```python
from build123d import *

# Parameters (mm, degrees)
F0_R         = 9.525
F1_DEPTH     = 25.4
F3_DEPTH     = 25.401
F4_DEPTH     = 11.0998
F6_DEPTH     = 5.08
F7_W         = 101.6
F7_H         = 127
F8_DEPTH     = 38.1
F9_T         = 2.54
F9_T3_DEPTH  = 10.16
F9_T5_DEPTH  = 11.43
F9_T7_DEPTH  = 11.43
F9_T9_DEPTH  = 11.43
F9_T11_DEPTH = 11.43
F9_T13_DEPTH = 11.43
F9_T15_DEPTH = 9.8425
F9_T17_DEPTH = 9.8425
F9_T19_DEPTH = 9.8425
F9_T21_DEPTH = 9.8425
F9_T23_DEPTH = 14.605
F9_T25_DEPTH = 16.1798
F9_T27_DEPTH = 14.605


# Not quite as in the source:
# - a shell that OpenCascade refuses in one call is made with other operations: the cavity is built on its own and cut out


with BuildPart() as f1:
    # F0 (on Front) → F1 (new body)
    with BuildSketch(Plane.XZ):
        Circle(F0_R)
    extrude(amount=F1_DEPTH)

    # F2 (on face) → F3 (cut, through all)
    with BuildSketch(Plane(origin=(0, 0, 0), x_dir=(-1, 0, 0), z_dir=(0, 1, 0))):
        with BuildLine():
            ThreePointArc((4.7625, 0), (3.3675960454, 3.3675960454), (0, 4.7625))
            ThreePointArc((0, 4.7625), (-3.3675960454, 3.3675960454), (-4.7625, 0))
            ThreePointArc((-4.7625, 0), (-3.3675960454, -3.3675960454), (0, -4.7625))
            ThreePointArc((0, -4.7625), (3.3675960454, -3.3675960454), (4.7625, 0))
        make_face()
    extrude(amount=-F3_DEPTH, mode=Mode.SUBTRACT)

    # F2 (on face) → F4 (cut)
    with BuildSketch(Plane(origin=(0, 0, 0), x_dir=(-1, 0, 0), z_dir=(0, 1, 0))):
        with BuildLine():
            Line((4.7625, 0), (4.7625, 4.7625))
            Line((4.7625, 4.7625), (0, 4.7625))
            ThreePointArc((0, 4.7625), (3.3675960454, 3.3675960454), (4.7625, 0))
        make_face()
        with BuildLine():
            ThreePointArc((-4.7625, 0), (-3.3675960454, 3.3675960454), (0, 4.7625))
            Line((0, 4.7625), (-4.7625, 4.7625))
            Line((-4.7625, 4.7625), (-4.7625, 0))
        make_face()
        with BuildLine():
            ThreePointArc((4.7625, 0), (3.3675960454, 3.3675960454), (0, 4.7625))
            ThreePointArc((0, 4.7625), (-3.3675960454, 3.3675960454), (-4.7625, 0))
            ThreePointArc((-4.7625, 0), (-3.3675960454, -3.3675960454), (0, -4.7625))
            ThreePointArc((0, -4.7625), (3.3675960454, -3.3675960454), (4.7625, 0))
        make_face()
        with BuildLine():
            Line((4.7625, -4.7625), (4.7625, 0))
            ThreePointArc((4.7625, 0), (3.3675960454, -3.3675960454), (0, -4.7625))
            Line((0, -4.7625), (4.7625, -4.7625))
        make_face()
        with BuildLine():
            ThreePointArc((0, -4.7625), (-3.3675960454, -3.3675960454), (-4.7625, 0))
            Line((-4.7625, 0), (-4.7625, -4.7625))
            Line((-4.7625, -4.7625), (0, -4.7625))
        make_face()
    extrude(amount=-F4_DEPTH, mode=Mode.SUBTRACT)

    # F5 (on face) → F6 (cut)
    with BuildSketch(Plane.XZ.offset(25.4)):
        Polygon((3.175, 5.499261314), (-3.175, 5.499261314), (-6.35, 0), (-3.175, -5.499261314), (3.175, -5.499261314), (6.35, 0), align=None)
    extrude(amount=-F6_DEPTH, mode=Mode.SUBTRACT)

    # F7 (on Front) → F8 (join)
    with BuildSketch(Plane.XZ):
        Rectangle(F7_W, F7_H)
    extrude(amount=-F8_DEPTH)

    # F9: shell of thickness 2.54, made by hand


with BuildPart() as f9_core1:
    # F9_t2: copy of F1
    add(f1.part)

    # the walls: a layer under each face that stays
    f9_faces = [f9_core1.faces().sort_by_distance(p)[0] for p in [
        (50.8, 19.05, 0),
        (0, 19.05, -63.5),
        (0, 19.05, 63.5),
        (-33.8666666667, 0, -42.3333333333),
        (-50.8, 19.05, 0),
        (-9.525, -12.7, 0),
        (-6.35, -25.4, -6.35),
        (0, -22.86, 5.499261314),
        (-4.7625, -22.86, 2.749630657),
        (-4.7625, -22.86, -2.749630657),
        (0, -22.86, -5.499261314),
        (4.7625, -22.86, -2.749630657),
        (4.7625, -22.86, 2.749630657),
        (-5.4428571429, -20.32, 0),
        (0, -15.7099, 4.7625),
        (-3.96875, -11.0998, -3.96875),
        (-3.96875, -11.0998, 3.96875),
        (3.96875, -11.0998, 3.96875),
        (3.96875, -11.0998, -3.96875),
        (-4.7625, -5.5499, 0),
        (0, -5.5499, -4.7625),
        (0, -5.5499, 4.7625),
        (4.7625, -5.5499, 0),
        (0, 0, 0),
    ]]
    thicken(f9_faces, amount=-F9_T, mode=Mode.SUBTRACT)

    # F9_s4 → F9_t3 (cut)
    with BuildSketch(Plane.XZ.offset(17.78)):
        Polygon((3.1530029547, 5.461161314), (3.175, 8.039261314), (4.6414696837, 8.039261314), (5.3747045256, 6.769261314), align=None)
        Polygon((-3.1530029547, 5.461161314), (-3.175, 8.039261314), (-4.6414696837, 8.039261314), (-5.3747045256, 6.769261314), align=None)
        Polygon((-6.3060059095, 0), (-8.5497045256, 1.27), (-9.2829393675, 0), (-8.5497045256, -1.27), align=None)
        Polygon((-3.1530029547, -5.461161314), (-5.3747045256, -6.769261314), (-4.6414696837, -8.039261314), (-3.175, -8.039261314), align=None)
        Polygon((3.1530029547, -5.461161314), (3.175, -8.039261314), (4.6414696837, -8.039261314), (5.3747045256, -6.769261314), align=None)
        Polygon((6.3060059095, 0), (8.5497045256, -1.27), (9.2829393675, 0), (8.5497045256, 1.27), align=None)
    extrude(amount=F9_T3_DEPTH, mode=Mode.SUBTRACT)

    # F9_s6 → F9_t5 (cut)
    with BuildSketch(Plane.YZ.offset(-5.715)):
        Polygon((-20.3454, 5.473861314), (-20.32, 8.039261314), (-17.78, 8.039261314), (-17.78, 5.499261314), align=None)
        Polygon((-20.3454, -5.473861314), (-20.32, -8.039261314), (-17.78, -8.039261314), (-17.78, -5.499261314), align=None)
    extrude(amount=F9_T5_DEPTH, mode=Mode.SUBTRACT)

    # F9_s8 → F9_t7 (cut)
    with BuildSketch(Plane(origin=(2.8575, 0, 4.9493351826), x_dir=(0, 1, 0), z_dir=(-0.5, 0, -0.8660254038))):
        Polygon((-20.3454, -5.473861314), (-20.32, -8.039261314), (-17.78, -8.039261314), (-17.78, -5.499261314), align=None)
    extrude(amount=F9_T7_DEPTH, mode=Mode.SUBTRACT)

    # F9_s10 → F9_t9 (cut)
    with BuildSketch(Plane(origin=(-2.8575, 0, 4.9493351826), x_dir=(0, 1, 0), z_dir=(0.5, 0, -0.8660254038))):
        Polygon((-20.3454, -5.473861314), (-20.32, -8.039261314), (-17.78, -8.039261314), (-17.78, -5.499261314), align=None)
    extrude(amount=F9_T9_DEPTH, mode=Mode.SUBTRACT)

    # F9_s12 → F9_t11 (cut)
    with BuildSketch(Plane(origin=(-2.8575, 0, -4.9493351826), x_dir=(0, 1, 0), z_dir=(0.5, 0, 0.8660254038))):
        Polygon((-20.3454, -5.473861314), (-20.32, -8.039261314), (-17.78, -8.039261314), (-17.78, -5.499261314), align=None)
    extrude(amount=F9_T11_DEPTH, mode=Mode.SUBTRACT)

    # F9_s14 → F9_t13 (cut)
    with BuildSketch(Plane(origin=(2.8575, 0, -4.9493351826), x_dir=(0, 1, 0), z_dir=(-0.5, 0, 0.8660254038))):
        Polygon((-20.3454, -5.473861314), (-20.32, -8.039261314), (-17.78, -8.039261314), (-17.78, -5.499261314), align=None)
    extrude(amount=F9_T13_DEPTH, mode=Mode.SUBTRACT)

    # F9_s16 → F9_t15 (cut)
    with BuildSketch(Plane.XY.offset(-7.3025)):
        Polygon((-4.7371, -11.0744), (-4.7625, -13.6398), (-7.3025, -13.6398), (-7.3025, -11.0998), align=None)
        Polygon((4.7371, -11.0744), (4.7625, -13.6398), (7.3025, -13.6398), (7.3025, -11.0998), align=None)
    extrude(amount=F9_T15_DEPTH, mode=Mode.SUBTRACT)

    # F9_s18 → F9_t17 (cut)
    with BuildSketch(Plane.YZ.offset(-7.3025)):
        Polygon((-11.0744, -4.7371), (-13.6398, -4.7625), (-13.6398, -7.3025), (-11.0998, -7.3025), align=None)
        Polygon((-11.0744, 4.7371), (-13.6398, 4.7625), (-13.6398, 7.3025), (-11.0998, 7.3025), align=None)
    extrude(amount=F9_T17_DEPTH, mode=Mode.SUBTRACT)

    # F9_s20 → F9_t19 (cut)
    with BuildSketch(Plane.XY.offset(-2.54)):
        Polygon((-4.7371, -11.0744), (-4.7625, -13.6398), (-7.3025, -13.6398), (-7.3025, -11.0998), align=None)
        Polygon((4.7371, -11.0744), (4.7625, -13.6398), (7.3025, -13.6398), (7.3025, -11.0998), align=None)
    extrude(amount=F9_T19_DEPTH, mode=Mode.SUBTRACT)

    # F9_s22 → F9_t21 (cut)
    with BuildSketch(Plane.YZ.offset(-2.54)):
        Polygon((-11.0744, 4.7371), (-13.6398, 4.7625), (-13.6398, 7.3025), (-11.0998, 7.3025), align=None)
        Polygon((-11.0744, -4.7371), (-13.6398, -4.7625), (-13.6398, -7.3025), (-11.0998, -7.3025), align=None)
    extrude(amount=F9_T21_DEPTH, mode=Mode.SUBTRACT)

    # F9_s24 → F9_t23 (cut)
    with BuildSketch(Plane.XY.offset(-7.3025)):
        Polygon((-4.7371, -0.0254), (-7.3025, 0), (-7.3025, 2.54), (-4.7625, 2.54), align=None)
        Polygon((4.7371, -0.0254), (7.3025, 0), (7.3025, 2.54), (4.7625, 2.54), align=None)
    extrude(amount=F9_T23_DEPTH, mode=Mode.SUBTRACT)

    # F9_s26 → F9_t25 (cut)
    with BuildSketch(Plane.XZ.offset(-2.54)):
        Polygon((-4.7371, -4.7371), (-7.3025, -4.7625), (-7.3025, -7.3025), (-4.7625, -7.3025), align=None)
        Polygon((-4.7371, 4.7371), (-7.3025, 4.7625), (-7.3025, 7.3025), (-4.7625, 7.3025), align=None)
        Polygon((4.7371, -4.7371), (4.7625, -7.3025), (7.3025, -7.3025), (7.3025, -4.7625), align=None)
        Polygon((4.7371, 4.7371), (4.7625, 7.3025), (7.3025, 7.3025), (7.3025, 4.7625), align=None)
    extrude(amount=F9_T25_DEPTH, mode=Mode.SUBTRACT)

    # F9_s28 → F9_t27 (cut)
    with BuildSketch(Plane.YZ.offset(-7.3025)):
        Polygon((-0.0254, -4.7371), (0, -7.3025), (2.54, -7.3025), (2.54, -4.7625), align=None)
        Polygon((-0.0254, 4.7371), (0, 7.3025), (2.54, 7.3025), (2.54, 4.7625), align=None)
    extrude(amount=F9_T27_DEPTH, mode=Mode.SUBTRACT)

    # F9_s29 → F9_t30 (revolve, cut)
    with BuildSketch(Plane.XY):
        Polygon((9.5504, -0.0254), (9.525, 2.54), (6.985, 2.54), (6.985, 0), align=None)
    revolve(axis=Axis((0, 0, 0), (0, -1, 0)), mode=Mode.SUBTRACT)


with BuildPart() as f1_1:
    add(f1.part)

    # what is left inside the walls is the cavity
    f9_cavity = [f9_core1.part.solids().sort_by_distance(p)[0] for p in [
        (0, 2.5654, -20.32),
    ]]
    add(f9_cavity, mode=Mode.SUBTRACT)


solid = f1_1.part
```
Input: part model. Units: mm. Frame: model coordinates. A direction names the side the tool comes from. Give positions to 0.01 mm unless a question says otherwise; leave off trailing zeros. Loops run counter-clockwise (first coordinate to the right, second up) from the corner with the lowest first, then second, coordinate; pieces in that order, holes last. Notation, with made-up numbers: (-31.75, 47.25) -> (11.25, 47.25) arc R21 ccw to (11.25, 80.25) -> close; hole circle Ø6 at (5, 14.5). An arc over 180 degrees is marked (long way). Use a Markdown table: item, result.
Q1. First-contact query: P1, Ø1, axis at x = -28.5, z = -6.5, coming from the +Y side; P2, Ø1.5, axis at x = -0.5, y = -23.5, coming from the -Z side (3 decimals); P3, Ø5.5, axis at x = 1, y = -22.5, coming from the +Z side (3 decimals). Flat tips, straight axial feed; report the tip coordinate or a pass-through.
Entries:
| item | result |
|---|---|
| P1 | stops at y = 2.54 |
| P2 | stops at z = -9.525 |
| P3 | stops at z = 9.525 |
Q2. Ray query, probe 1 along Z at (x, y) = (-11, 35); probe 2 along X at (y, z) = (16, 32.5); probe 3 along Y at (x, z) = (45.5, 39). Return the intervals inside material, ascending. Write a range as from..to.
Entries:
| item | result |
|---|---|
| probe 1 | z = -63.5..-60.96, 60.96..63.5 |
| probe 2 | x = -50.8..-48.26, 48.26..50.8 |
| probe 3 | y = 0..2.54 |
Q3. Access query for faces 1 (the flat face through (-1, 19, 63.5)), 2 (the flat face through (48.26, 20, -1)), 3 (the flat face through (-4, -11.1, 4)), 4 (the flat face through (-1, 19, -63.5)). Directions: +Z, -Z, +X, -X, +Y, -Y. A direction counts if a zero-diameter tool reaches every point of the face in a straight line with its end or side. Return the directions, or none.
Entries:
| item | result |
|---|---|
| face 1 | +Z, +X, -X, +Y, -Y |
| face 2 | +Y |
| face 3 | none |
| face 4 | -Z, +X, -X, +Y, -Y |
Q4. Section query B-B, the plane z = -38.5. Return the cut outline in (x, y).
Entries:
| item | result |
|---|---|
| outline | (-50.8, 0) -> (50.8, 0) -> (50.8, 38.1) -> (48.26, 38.1) -> (48.26, 2.54) -> (-48.26, 2.54) -> (-48.26, 38.1) -> (-50.8, 38.1) -> close |
Q5. Section query A-A, the plane y = 12. Return the cut outline in (x, z), plus the area to 3 significant figures.
Entries:
| item | result |
|---|---|
| outline | (-50.8, -63.5) -> (50.8, -63.5) -> (50.8, 63.5) -> (-50.8, 63.5) -> close; hole (-48.26, -60.96) -> (48.26, -60.96) -> (48.26, 60.96) -> (-48.26, 60.96) -> close |
| area | 1,140 mm² |
Q6. Section query C-C, the plane x = -21.5. Return the cut outline in (y, z).
Entries:
| item | result |
|---|---|
| outline | (0, -63.5) -> (38.1, -63.5) -> (38.1, -60.96) -> (2.54, -60.96) -> (2.54, 60.96) -> (38.1, 60.96) -> (38.1, 63.5) -> (0, 63.5) -> close |
Q7. Section query D-D, the plane z = -8. Return the cut outline in (x, y).
Entries:
| item | result |
|---|---|
| outline | (-50.8, 0) -> (-5.17, 0) -> (-5.17, -25.4) -> (5.17, -25.4) -> (5.17, 0) -> (50.8, 0) -> (50.8, 38.1) -> (48.26, 38.1) -> (48.26, 2.54) -> (-48.26, 2.54) -> (-48.26, 38.1) -> (-50.8, 38.1) -> close |
Q8. Pull-direction query (X, two-part tool) for faces 5 (the flat face through (4.74, -22.9, -2.79)), 6 (the flat face through (-4.4, -25.4, -4.1)); classes: pulls with the +X half, pulls with the -X half, needs draft (parallel to the pull), parting line crosses it, or undercut.
Entries:
| item | result |
|---|---|
| face 5 | undercut |
| face 6 | needs draft |
